Work out the finished part from the listing and answer in its coordinate system (mm). Give positions to 0.01 mm unless a question says otherwise; leave off trailing zeros. Order: outer loops, then holes, each group sorted by start corner. A loop starts at its lowest first (then second) coordinate and runs counter-clockwise, first axis right, second up. Notation, with made-up numbers: (38, 89) - (55, 89) arc R12 ccw to (55, 111) - close; hole circle Ø3 at (88.25, 28.25). An arc over 180 degrees is marked (long way). Write each question's results on one line, items separated by ' | '.
from build123d import *

# Parameters (mm, degrees)
F4_R     = 3.175
F5_DEPTH = 50.8


with BuildPart() as f2:
    # F0 (on Front) → F2 (revolve)
    with BuildSketch(Plane.XZ):
        with BuildLine():
            Line((0, -9.525), (0, 9.525))
            ThreePointArc((0, 9.525), (-9.525, 0), (0, -9.525))
        make_face()
    revolve(axis=Axis((0, 0, 0), (0, 0, 1)))


with BuildPart() as f5:
    # F4 (on offset) → F5 (new body)
    with BuildSketch(Plane.XY.offset(6.35)):
        Circle(F4_R)
    extrude(amount=F5_DEPTH)

    # F6: cut F2
    add(f2.part, mode=Mode.SUBTRACT)


solid = f5.part
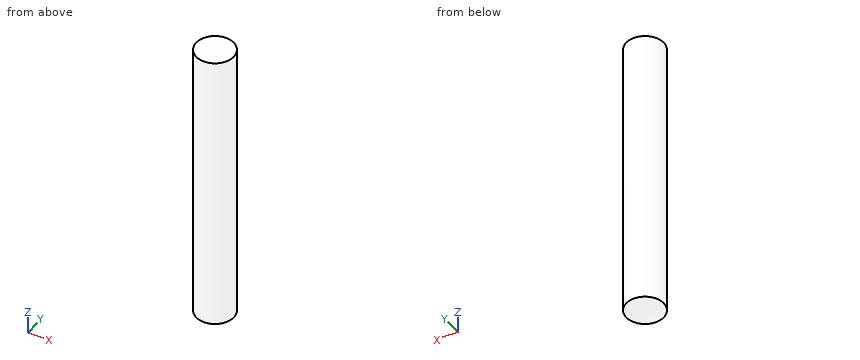
1. A cutting plane is placed at C-C, the plane y = -0.75. Write down the section's boundary in (x, z), then the cut area to 3 significant figures.
Answer list:
outline: (-3.09, 8.98) arc R9.5 cw to (3.09, 8.98) - (3.09, 57.15) - (-3.09, 57.15) - close | area: 295 mm^2
2. A cutting plane is placed at B-B, the plane x = -1. Write down the section's boundary in (y, z), then the cut area to 3 significant figures.
Answer list:
outline: (-3.01, 8.98) arc R9.47 cw to (3.01, 8.98) - (3.01, 57.15) - (-3.01, 57.15) - close | area: 288 mm^2
3. A cutting plane is placed at A-A, the plane z = 23. Write down the section's boundary in (x, y) (3 decimals).
Answer list:
outline: circle Ø6.35 at (0, 0)
4. Straight lines are drawn through the part: line 1 (Z direction, x = -0.25, y = -0.25); line 2 (Y direction, x = 1.25, z = 25); line 3 (X direction, y = -2.5, z = 21). For each, find the intervals that lie inside material, in ascending order. Write a range as [from, to].
Answer list:
line 1: [9.52, 57.15] | line 2: [-2.92, 2.92] | line 3: [-1.96, 1.96]
